from build123d import *

# Parameters (mm, degrees)
SKETCH2_R           = 20
SKETCH2_R_2         = 5
BOSS_EXTRUDE1_DEPTH = 10
BOSS_EXTRUDE2_DEPTH = 3
CIRPATTERN1_COUNT   = 2
SKETCH5_R           = 2.5
BOSS_EXTRUDE3_DEPTH = 5
BOSS_EXTRUDE4_START = 5
SKETCH6_R           = 2.5
BOSS_EXTRUDE4_DEPTH = 5
CUT_EXTRUDE1_DEPTH  = 147
FILLET1_R           = 2
SKETCH8_R           = 11.27429685
BOSS_EXTRUDE5_DEPTH = 3
FILLET2_R           = 5
SKETCH9_R           = 11.275
BOSS_EXTRUDE6_DEPTH = 3
FILLET3_R           = 5


with BuildPart() as part:
    # Sketch2 → Boss-Extrude1 (new body)
    with BuildSketch(Plane.XY):
        Circle(SKETCH2_R)
        Circle(SKETCH2_R_2, mode=Mode.SUBTRACT)
    extrude(amount=BOSS_EXTRUDE1_DEPTH)

    # Sketch4 → Boss-Extrude2 (add)
    with BuildSketch(Plane(origin=(20, 0, 0), x_dir=(0, 0, -1), z_dir=(1, 0, 0))):
        with BuildLine():
            Line((-82.207951234, 19.918138143), (-19.990870076, 19.918138143))
            ThreePointArc((-19.990870076, 19.918138143), (-9.096212625, 16.67449148), (-1.749920893, 8))
            Line((-1.749920893, 8), (-10, 8))
            Line((-10, 8), (-10, -8))
            Line((-10, -8), (-1.749920893, -8))
            ThreePointArc((-1.749920893, -8), (-9.096212625, -16.67449148), (-19.990870076, -19.918138143))
            Line((-19.990870076, -19.918138143), (-82.207951234, -19.918138143))
            ThreePointArc((-82.207951234, -19.918138143), (-102.126089377, 0), (-82.207951234, 19.918138143))
        make_face()
    boss_extrude2 = extrude(amount=-BOSS_EXTRUDE2_DEPTH)

    # CirPattern1: Boss-Extrude2 ×2 about axis
    cirpattern1_axis = Axis((0, 0, 0), (0, 0, 1))
    for i in range(1, CIRPATTERN1_COUNT):
        add(boss_extrude2.rotate(cirpattern1_axis, i * 360 / CIRPATTERN1_COUNT))

    # Sketch5 → Boss-Extrude3 (add)
    with BuildSketch(Plane(origin=(-17, 0, 0), x_dir=(0, 0, -1), z_dir=(1, 0, 0))):
        with Locations(Location((-82.207951234, 0, 0), (0, 0, 180))):
            Circle(SKETCH5_R)
    extrude(amount=BOSS_EXTRUDE3_DEPTH)

    # Sketch6 → Boss-Extrude4 (add)
    with BuildSketch(Plane.ZY.offset(-17).offset(BOSS_EXTRUDE4_START)):
        with Locations((82.207951234, 0)):
            Circle(SKETCH6_R)
    extrude(amount=-BOSS_EXTRUDE4_DEPTH)

    # Sketch7 → Cut-Extrude1 (cut)
    with BuildSketch(Plane(origin=(20, 0, 0), x_dir=(0, 0, -1), z_dir=(1, 0, 0))):
        with BuildLine():
            Line((-82.207951234, 19.918138143), (-19.990870076, 19.918138143))
            ThreePointArc((-19.990870076, 19.918138143), (-51.099410655, 12.742712192), (-82.207951234, 19.918138143))
        make_face()
        with BuildLine():
            Line((-82.207951234, -19.918138143), (-19.990870076, -19.918138143))
            ThreePointArc((-19.990870076, -19.918138143), (-51.099410655, -12.873612926), (-82.207951234, -19.918138143))
        make_face()
    extrude(amount=-CUT_EXTRUDE1_DEPTH, mode=Mode.SUBTRACT)

    # Fillet1
    # the kernel refuses this fillet: 2 mm, written as the material it takes off along each edge
    with BuildSketch(Plane(origin=(-20, -85.083350362, 51.099410655), x_dir=(0, 0.8704701074712403, -0.49222128356970424), z_dir=(0, -0.49222128356970424, -0.8704701074712403))) as fillet1_piece_1:
        with BuildLine():
            CenterArc((72.209737436 + FILLET1_R, FILLET1_R), FILLET1_R, 180, 90)
            Line((72.209737436 + FILLET1_R, 0), (72.209737436, 0))
            Line((72.209737436, 0), (72.209737436, FILLET1_R))
        make_face()
    revolve(axis=Axis((-20, -85.083350362, 51.099410655), (1, 0, 0)), revolution_arc=58.973369899, mode=Mode.SUBTRACT)
    with BuildSketch(Plane(origin=(-17, -85.083350362, 51.099410655), x_dir=(0, 0.8704701074712403, -0.49222128356970424), z_dir=(0, -0.49222128356970424, -0.8704701074712403))) as fillet1_piece_2:
        with BuildLine():
            CenterArc((72.209737436 + FILLET1_R, -FILLET1_R), FILLET1_R, 90, 90)
            Line((72.209737436, -FILLET1_R), (72.209737436, 0))
            Line((72.209737436, 0), (72.209737436 + FILLET1_R, 0))
        make_face()
    revolve(axis=Axis((-17, -85.083350362, 51.099410655), (1, 0, 0)), revolution_arc=58.973369899, mode=Mode.SUBTRACT)
    with BuildSketch(Plane(origin=(-17, 83.764839764, 51.099410655), x_dir=(0, -0.8659267657003706, 0.5001708072685723), z_dir=(0, 0.5001708072685723, 0.8659267657003706))) as fillet1_piece_3:
        with BuildLine():
            CenterArc((71.022127572 + FILLET1_R, -FILLET1_R), FILLET1_R, 90, 90)
            Line((71.022127572, -FILLET1_R), (71.022127572, 0))
            Line((71.022127572, 0), (71.022127572 + FILLET1_R, 0))
        make_face()
    revolve(axis=Axis((-17, 83.764839764, 51.099410655), (1, 0, 0)), revolution_arc=60.022602323, mode=Mode.SUBTRACT)
    with BuildSketch(Plane(origin=(-20, 83.764839764, 51.099410655), x_dir=(0, -0.8659267657003706, 0.5001708072685723), z_dir=(0, 0.5001708072685723, 0.8659267657003706))) as fillet1_piece_4:
        with BuildLine():
            CenterArc((71.022127572 + FILLET1_R, FILLET1_R), FILLET1_R, 180, 90)
            Line((71.022127572 + FILLET1_R, 0), (71.022127572, 0))
            Line((71.022127572, 0), (71.022127572, FILLET1_R))
        make_face()
    revolve(axis=Axis((-20, 83.764839764, 51.099410655), (1, 0, 0)), revolution_arc=60.022602323, mode=Mode.SUBTRACT)
    with BuildSketch(Plane(origin=(17, 83.764839764, 51.099410655), x_dir=(0, -0.8659267657003706, 0.5001708072685723), z_dir=(0, 0.5001708072685723, 0.8659267657003706))) as fillet1_piece_5:
        with BuildLine():
            CenterArc((71.022127572 + FILLET1_R, FILLET1_R), FILLET1_R, 180, 90)
            Line((71.022127572, FILLET1_R), (71.022127572, 0))
            Line((71.022127572, 0), (71.022127572 + FILLET1_R, 0))
        make_face()
    revolve(axis=Axis((17, 83.764839764, 51.099410655), (1, 0, 0)), revolution_arc=60.022602323, mode=Mode.SUBTRACT)
    with BuildSketch(Plane(origin=(20, -85.083350362, 51.099410655), x_dir=(0, 0.8704701074712403, -0.49222128356970424), z_dir=(0, -0.49222128356970424, -0.8704701074712403))) as fillet1_piece_6:
        with BuildLine():
            CenterArc((72.209737436 + FILLET1_R, -FILLET1_R), FILLET1_R, 90, 90)
            Line((72.209737436, -FILLET1_R), (72.209737436, 0))
            Line((72.209737436, 0), (72.209737436 + FILLET1_R, 0))
        make_face()
    revolve(axis=Axis((20, -85.083350362, 51.099410655), (1, 0, 0)), revolution_arc=58.973369899, mode=Mode.SUBTRACT)
    with BuildSketch(Plane(origin=(20, 83.764839764, 51.099410655), x_dir=(0, -0.8659267657003705, -0.5001708072685725), z_dir=(0, 0.5001708072685725, -0.8659267657003705))) as fillet1_piece_7:
        with BuildLine():
            CenterArc((71.022127572 + FILLET1_R, FILLET1_R), FILLET1_R, 180, 90)
            Line((71.022127572, FILLET1_R), (71.022127572, 0))
            Line((71.022127572, 0), (71.022127572 + FILLET1_R, 0))
        make_face()
    revolve(axis=Axis((20, 83.764839764, 51.099410655), (-1, 0, 0)), revolution_arc=60.022602323, mode=Mode.SUBTRACT)

    # Sketch8 → Boss-Extrude5 (add)
    with BuildSketch(Plane(origin=(20, 0, 0), x_dir=(0, 0, -1), z_dir=(1, 0, 0))):
        with Locations((-82.207951234, 0)):
            Circle(SKETCH8_R)
    extrude(amount=BOSS_EXTRUDE5_DEPTH)

    # Fillet2
    # the kernel refuses this fillet: 5 mm, written as the material it takes off along each edge
    with BuildSketch(Plane(origin=(23, 0, 82.207951234), x_dir=(0, 0, -1), z_dir=(0, -1, 0))) as fillet2_piece_1:
        with BuildLine():
            CenterArc((6.691721155, -5), FILLET2_R, 23.578178478, 66.421821522)
            Line((6.691721155, 0), (6.691721155, 0.1))
            Line((6.691721155, 0.1), (11.27429685, 0.1))
            Line((11.27429685, 0.1), (11.37429685, 0))
            ThreePointArc((11.37429685, 0), (11.37429685, -1.5), (11.365948364, -2.96))
            Line((11.365948364, -2.96), (11.27429685, -3))
        make_face()
    revolve(axis=Axis((23, 0, 82.207951234), (1, 0, 0)), mode=Mode.SUBTRACT)

    # Sketch9 → Boss-Extrude6 (add)
    with BuildSketch(Plane.ZY.offset(20)):
        with Locations((82.207951234, 0)):
            Circle(SKETCH9_R)
    extrude(amount=BOSS_EXTRUDE6_DEPTH)

    # Fillet3
    # the kernel refuses this fillet: 5 mm, written as the material it takes off along each edge
    with BuildSketch(Plane(origin=(-23, 0, 82.207951234), x_dir=(0, 0, 1), z_dir=(0, -1, 0))) as fillet3_piece_1:
        with BuildLine():
            CenterArc((6.692424305, -5), FILLET3_R, 23.578178478, 66.421821522)
            Line((6.692424305, 0), (6.692424305, 0.1))
            Line((6.692424305, 0.1), (11.275, 0.1))
            Line((11.275, 0.1), (11.375, 0))
            ThreePointArc((11.375, 0), (11.375, -1.5), (11.366651514, -2.96))
            Line((11.366651514, -2.96), (11.275, -3))
        make_face()
    revolve(axis=Axis((-23, 0, 82.207951234), (-1, 0, 0)), mode=Mode.SUBTRACT)


solid = part.part
Verification items for the finished model (mm, model axes). A direction names the side the tool comes from. Coordinates: 2 decimals unless noted, no trailing zeros. Write each loop counter-clockwise with the first axis right and the second up, starting at its lowest first coordinate (ties: lowest second). Pieces come first, ordered by that corner, then holes. Notation, with made-up numbers: (4, 45.5) -> (17, 45.5) arc R10 ccw to (17, 53.5) -> close; hole circle Ø4 at (0.5, 56.5). An arc over 180 degrees is marked (long way). One line per item, written item: value. Start each with the question number.
Q1. Go/stop test with flat-tipped pins: P1, Ø1.5, axis at y = -5.5, z = 58.5, coming from the -X side; P2, Ø10, axis at x = -13, z = 41, coming from the -Y side; P3, Ø2, axis at y = -15.5, z = 91, coming from the +X side. Record where each tip stops, or that it passes through.
Q2. Cross-section at C-C on x = 13. Enter the section's corners in (y, z).
Q3. Cross-section at A-A on x = 0. Enter the section's corners in (y, z), and give its area (3 significant figures).
Q4. Mould release check, pull along Y, two halves, no side actions. Record for faces 1 (the cylindrical face through (17.507, -12.875, 50.649)), 2 (the flat face through (-12, 0, 82)), 3 (the cylindrical face through (-1.08, -4.88, 4.93)), 4 (the cylindrical face through (-4.336, -19.524, 4.93)): pulls with the +Y half, pulls with the -Y half, needs draft (parallel to the pull), parting line crosses it, or undercut.
Q5. Cross-section at B-B on y = 16. State how many separate pieces and enclosed holes the cut face has, and give its area (3 significant figures).
Q6. Thickness scan on L1, parallel to X at y = 13, z = 29; L2, parallel to X at y = 2.5, z = 77.5; L3, parallel to Y at x = 0, z = 3. Record the ranges inside material, lowest first. Write a range as from..to.
Q7. Access from +Z, -Z, +X, -X, +Y, -Y to the whole of each face (thin tool, end or side, straight path). Record for faces 5 (the cylindrical face through (-14.54, -0.11, 79.71)), 6 (the flat face through (12, 0, 82)), 7 (the cylindrical face through (18.521, 16.723, 9.17)).
Checked values:
1. P1: stops at x = -20
1. P2: stops at y = -13.4
1. P3: stops at x = 20
2. outline: (-15.2, 0) -> (15.2, 0) -> (15.2, 10) -> (-15.2, 10) -> close; circle Ø5 at (0, 82.21)
3. outline: (-20, 0) -> (-5, 0) -> (-5, 10) -> (-20, 10) -> close; (5, 0) -> (20, 0) -> (20, 10) -> (5, 10) -> close
3. area: 300 mm²
4. face 1: pulls with the -Y half
4. face 2: needs draft
4. face 3: undercut
4. face 4: undercut
5. separate pieces: 5
5. enclosed holes: 0
5. area: 479 mm²
6. L1: x = -20..-17, 17..20
6. L2: x = -23..-17, 17..23
6. L3: y = -20..-5, 5..20
7. face 5: none
7. face 6: +Z, +Y, -Y
7. face 7: -Z, +X, +Y
